Autodesk Inventor part; units mm, degrees
ref_plane "YZ Plane" through (0, 0, 0) normal (1, 0, 0) x (0, 1, 0)
ref_plane "XZ Plane" through (0, 0, 0) normal (0, 1, 0) x (-1, 0, 0)
ref_plane "XY Plane" through (0, 0, 0) normal (0, 0, 1) x (1, 0, 0)
sketch "Sketch1" plane through (0, 0, 0) normal (0, 1, 0) x (-1, 0, 0)
  line L0 (0, 0) -> (-33, 0) construction
  line L1 (-6.5, 6.5) -> (-26.5, 6.5)
  line L2 (-26.5, -6.5) -> (-6.5, -6.5)
  arc A0 (-6.5, -6.5) -> (-6.5, 6.5) centre (-6.5, 0) ccw
  arc A1 (-26.5, 6.5) -> (-26.5, -6.5) centre (-26.5, 0) ccw
  circle A2 centre (-6.5, 0) radius 2
  line L3 (-22.6527, -1.0329) -> (-22.6527, 4.8111) construction
  line L4 (-22.6527, 4.8111) -> (-19.4837, 4.8111) construction
  line L5 (-19.4837, 4.8111) -> (-19.4837, -1.0329) construction
  line L6 (-19.4837, -1.0329) -> (-22.6527, -1.0329) construction
  line L7 (-26.5, 0) -> (-33, 0) construction
  line L8 (-26.5, -6.5) -> (-26.5, 6.5)
  line L9 (-33, 0) -> (-16.5, 0) construction
  line L10 (-32, -1) -> (-17.5, -1)
  line L11 (-17.5, 1) -> (-32, 1)
  arc A3 (-32, 1) -> (-32, -1) centre (-32, 0) ccw
  arc A4 (-17.5, -1) -> (-17.5, 1) centre (-17.5, 0) ccw
  line L12 (-22.6527, 0.0867) -> (-19.5369, 0.0867)
  line L13 (-19.5369, 0.0867) -> (-19.5369, -0.1112)
  line L14 (-19.5369, -0.1112) -> (-22.3445, -0.1112)
  spline S0 degree 2 poles (-22.3445, -0.1112) (-22.2032, -0.2582) (-21.9996, -0.6343) (-21.9204, -0.8576) knots 0 0 0 1 2 2 2
  line L15 (-21.9204, -0.8576) -> (-22.0985, -0.8576)
  spline S1 degree 2 poles (-22.0985, -0.8576) (-22.1438, -0.7219) (-22.2569, -0.4929) (-22.3926, -0.2836) (-22.5566, -0.0857) (-22.6527, 0.0161) knots 0 0 0 1 2 3 4 4 4
  line L16 (-22.6527, 0.0161) -> (-22.6527, 0.0867)
  point P0 (-29.75, 0)
  point P1 (-24.75, 0)
  point P2 (-26.5, -1)
  point P3 (-26.5, 1)
  dimension "d0" = 33
  dimension "d1" = 13
  dimension "d2" = 4
  dimension "d18" = 2
  dimension "d19" = 5.5
extrude "Plate1" add sketch "Sketch1" against normal blind 0.45 contours A0 L2 L8 L10 A4 L11 L1 | A3 L11 L8 L10 | L11 A4 L10 L8 | A2 | L12 L13 L14 S0 L15 S1 L16
hole "Hole1" at (6.5, 0, 0) direction (0, -1, 0) diameter 4.4958 end through all
emboss "Emboss2" sketch "Sketch1" operation cut depth 0.01 direction (0, -1, 0) draft 45 contours L12 L13 L14 S0 L15 S1 L16
fillet "Fillet1" radius 1 2 edges at (26.5, -0.225, 6.5) (26.5, -0.225, -6.5)
fillet "Fillet3" radius 5.5 2 edges at (26.5, -0.225, 1) (26.5, -0.225, -1)
equation "\"d9\" = Thickness"
equation "\"d20\" = d19"
equation "\"d3\" = Thickness"
equation "\"BendRadius\" = Thickness"
equation "\"BendReliefWidth\" = Thickness"
equation "\"BendReliefDepth\" = 0.5 * Thickness"
equation "\"CornerReliefSize\" = 4 * Thickness"
equation "\"MinimumRemnant\" = 2 * Thickness"
equation "\"TransitionRadius\" = BendRadius"
equation "\"JacobiRadiusSize\" = BendRadius"
equation "\"GapSize\" = Thickness"
properties part number "Part16.5mm" material "Steel, Carbon"
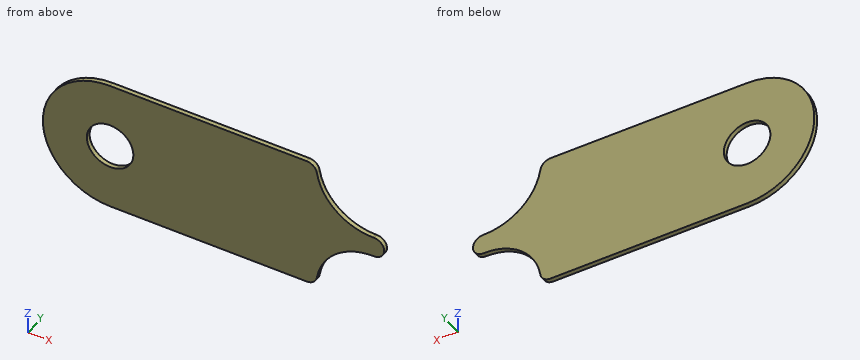
CAD build for the part. Positions are in the model's coordinates, mm. Round coordinates to 2 decimals unless told otherwise and drop trailing zeros. Loops run counter-clockwise (first coordinate to the right, second up) from the corner with the lowest first, then second, coordinate; pieces in that order, holes last.
(1) Drop flat-ended pins along their axis: pin 1 (4 mm diameter, centred on x = 9, z = 4, fed in from +Y); pin 2 (4 mm diameter, centred on x = 6.5, z = 0, fed in from -Y). Give the stop position or say it passes through.
(2) Cut at A-A (z = 0). Give the cut face in (x, y), plus the area to 3 significant figures.
(3) Wall check: line 1 along Z through (x, y) = (6.5, -0.1); line 2 along X through (y, z) = (-0.15, 0); line 3 along X through (y, z) = (-0.3, -2). Give the ranges that are in metal, low to high.
Findings below:
1. pin 1: stops at y = 0
1. pin 2: passes through
2. outline: (0, -0.45) - (4.25, -0.45) - (4.25, 0) - (0, 0) - close; (8.75, -0.45) - (33, -0.45) - (33, 0) - (8.75, 0) - close
2. area: 12.8 mm2
3. line 1: z = -6.5 to -2.25, 2.25 to 6.5
3. line 2: x = 0 to 4.25, 8.75 to 33
3. line 3: x = 0.32 to 5.47, 7.53 to 28.76
